Part print with two shaded views. Sizes in mm from the minimum x, y, z corner. Coordinates: 2 decimals unless noted, no trailing zeros. Write each loop counter-clockwise with the first axis right and the second up, starting at its lowest first coordinate (ties: lowest second). Pieces come first, ordered by that corner, then holes. Notation, with made-up numbers: (22, -32.75) - (79, -32.75) arc R22 ccw to (79, -15.75) - close; hole circle Ø8 at (59.25, 80.25). An arc over 180 degrees is marked (long way). Answer in a Markdown table with one row per item. Add a question column.
Q1. Band-saw the part on A-A (y = 50). State how many separate pieces and enclosed holes the cut face has, and give its area (3 significant figures).
Q2. Band-saw the part on B-B (z = 27.5). List the corners of the cut face in (x, y).
Q3. Drill centre lines: line 1 along X through (y, z) = (37, 10) (1 decimal); line 2 along Z through (x, y) = (100, 44) (1 decimal); line 3 along Z through (x, y) = (28, 18.5) (1 decimal). Where is each one in solid material? Low to high. Write a range as from..to.
Q4. Pin check, flat tips, straight feed: pin 1 (12 mm diameter, centred on x = 107, y = 41.5, fed in from +Z); pin 2 (1.9 mm diameter, centred on x = 100, z = 10, fed in from -Y). Stop position of each tip, or through.
Q5. Band-saw the part on C-C (x = 30). List the corners of the cut face in (y, z).
Q6. Two-plate mould, pull along Z, no slides. Class the marked faces 1, 2 and 3: +Z half, -Z half, draft (parallel to the pull), parting line (faces both ways), or undercut.
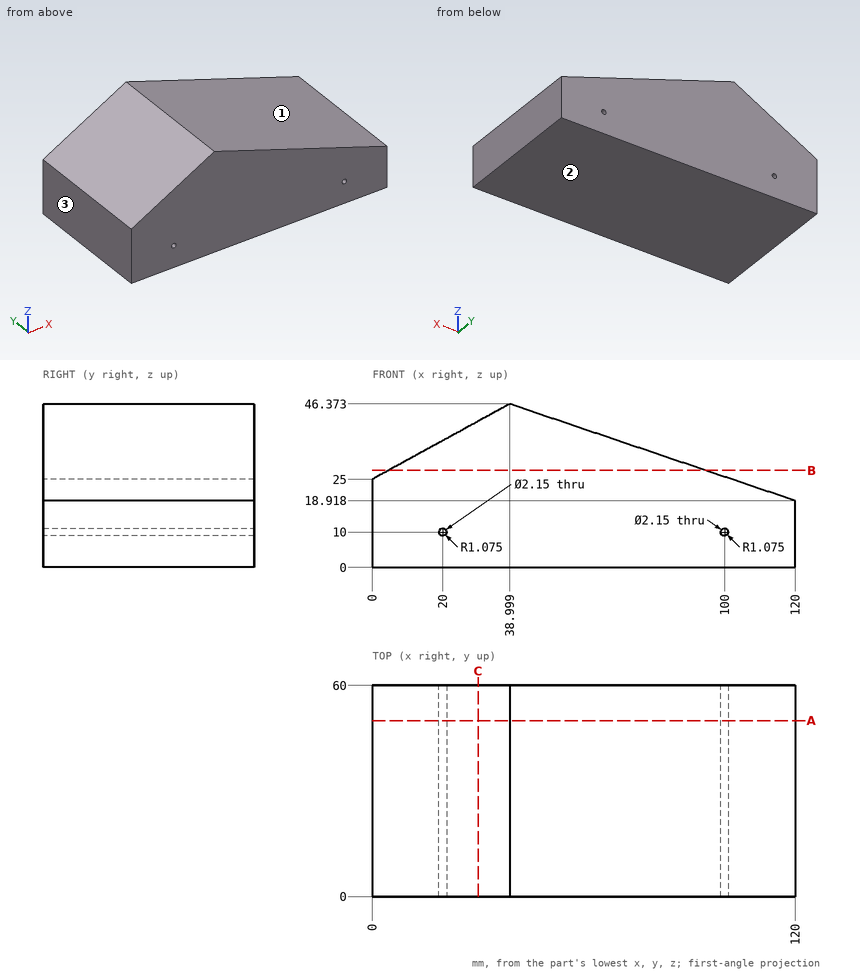
Checked values:
| question | item | result |
|---|---|---|
| 1 | separate pieces | 1 |
| 1 | enclosed holes | 2 |
| 1 | area | 4,030 mm² |
| 2 | outline | (4.56, 0) - (94.68, 0) - (94.68, 60) - (4.56, 60) - close |
| 3 | line 1 | x = 0..18.9, 21.1..98.9, 101.1..120 |
| 3 | line 2 | z = 0..8.9, 11.1..25.7 |
| 3 | line 3 | z = 0..40.3 |
| 4 | pin 1 | stops at z = 25.36 |
| 4 | pin 2 | passes through |
| 5 | outline | (0, 0) - (60, 0) - (60, 41.44) - (0, 41.44) - close |
| 6 | face 1 | +Z half |
| 6 | face 2 | -Z half |
| 6 | face 3 | draft |
